Answer from the drawing. Dimensions are ordinates in mm from the lowest x, y and z of the part. Give positions to 0.01 mm unless a question says otherwise; leave off trailing zeros. Order: outer loops, then holes, each group sorted by start corner. A loop starts at its lowest first (then second) coordinate and runs counter-clockwise, first axis right, second up. Notation, with made-up numbers: M 58,-13.75 L 87,-13.75 A15 ccw 87,11.25 Z; hole C 2,40 d9. An arc over 180 degrees is marked long. One line per item, written item: value.
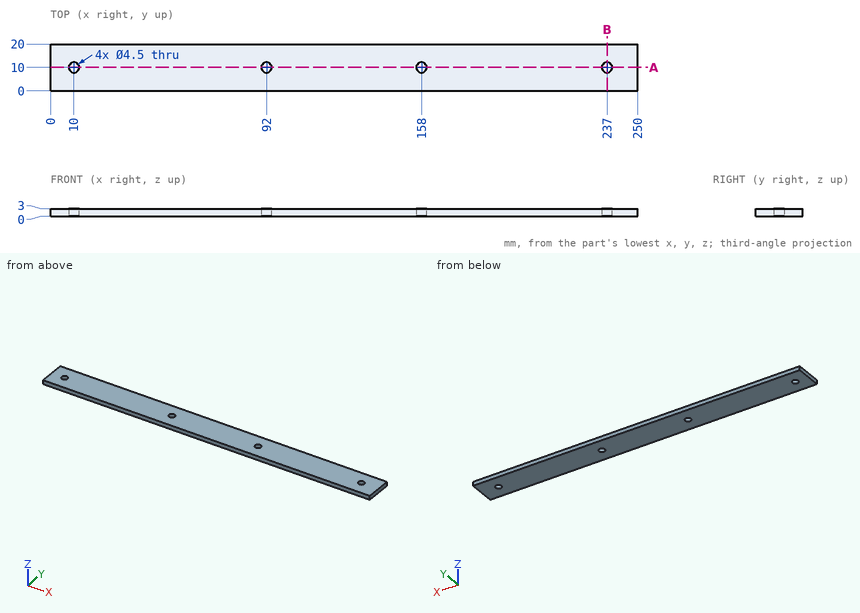
(1) Given P1, Ø12, axis at x = 93, y = 18, coming from the -Z side, flat-ended and moving along its own axis, determine where the tip first touches the part or whether it passes through.
Findings:
P1: stops at z = 0
(2) Section B-B, the plane x = 237 is taken. Give the vertices of the cut face in (y, z).
Findings:
outline: M 0,0 L 7.75,0 L 7.75,3 L 0,3 Z; M 12.25,0 L 20,0 L 20,3 L 12.25,3 Z
(3) Section A-A, the plane y = 10 is taken. Give the vertices of the cut face in (x, z), then the cut area to 3 significant figures.
Findings:
outline: M 0,0 L 7.75,0 L 7.75,3 L 0,3 Z; M 12.25,0 L 89.75,0 L 89.75,3 L 12.25,3 Z; M 94.25,0 L 155.75,0 L 155.75,3 L 94.25,3 Z; M 160.25,0 L 234.75,0 L 234.75,3 L 160.25,3 Z; M 239.25,0 L 250,0 L 250,3 L 239.25,3 Z
area: 696 mm^2
(4) Find the intervals of material crossed by probe 1 along X at (y, z) = (9, 1.05); probe 2 along Y at (x, z) = (158, 1.8); probe 3 along X at (y, z) = (11.5, 2.9), in increasing order. Write a range as from..to.
Findings:
probe 1: x = 0..7.98, 12.02..89.98, 94.02..155.98, 160.02..234.98, 239.02..250
probe 2: y = 0..7.75, 12.25..20
probe 3: x = 0..8.32, 11.68..90.32, 93.68..156.32, 159.68..235.32, 238.68..250
